Autodesk Inventor part; units mm, degrees
ref_plane "Work Plane1" through (0, 5, 0) normal (0, 1, 0) x (1, 0, 0)
ref_plane "YZ Plane" through (0, 0, 0) normal (1, 0, 0) x (0, 1, 0)
ref_plane "XZ Plane" through (0, 0, 0) normal (0, 1, 0) x (-1, 0, 0)
sketch "Sketch1" plane through (0, 0, 0) normal (0, 1, 0) x (-1, 0, 0)
  line L0 (0, -10) -> (-8.6603, -5)
  line L1 (-8.6603, -5) -> (-8.6603, 5)
  line L2 (-8.6603, 5) -> (0, 10)
  line L3 (0, 10) -> (8.6603, 5)
  line L4 (8.6603, 5) -> (8.6603, -5)
  line L5 (8.6603, -5) -> (0, -10)
  point P0 (0, 0)
  point P1 (0, 0)
  dimension "d1" = 20
extrude "Extrusion1" add sketch "Sketch1" along normal blind 10
sketch "Sketch2" plane through (0, 0, 0) normal (1, 0, 0) x (0, 1, 0)
  line L0 (10, -5) -> (10, -10)
  line L1 (10, -10) -> (8.5, -10)
  line L2 (10, -8.5) -> (10, -10)
  line L3 (8.5, -10) -> (10, -8.5)
  line L4 (-2, 0) -> (12, 0)
  point P0 (0, 0)
revolve "Revolution1" cut sketch "Sketch2" angle 360 about axis through (0, -10, 0) along (0, 1, 0)
ref_plane "Work Plane1" through (0, 5, 0) normal (0, 1, 0) x (1, 0, 0)
mirror "Mirror1" about plane through (0, 5, 0) normal (0, 1, 0) of "Revolution1"
sketch "Sketch3" plane through (0, 10, 0) normal (0, 1, 0) x (1, 0, 0)
  circle A0 centre (0, 0) radius 8.5
hole "Hole1" at (0, 10, 0) direction (0, -1, 0) diameter 10.917 depth 29.1 tip angle 118
chamfer "Chamfer1" distance 0.5 angle 45 2 edges at (0, 10, -5.4585) (0, 0, -5.4585)
properties part number "nut"
Could you check a few things on this model? Use its own coordinates, in mm. Give positions to 0.01 mm unless a question says otherwise; leave off trailing zeros. Order: outer loops, then holes, each group sorted by start corner. A loop starts at its lowest first (then second) coordinate and runs counter-clockwise, first axis right, second up. Notation, with made-up numbers: (83.25, 70) -> (117.25, 70) arc R28 cw to (117.25, 109) -> close; hole circle Ø2 at (43, -31). An arc over 180 degrees is marked (long way). Return JSON: item names as keys, results as strings.
1. Imagine slicing it at B-B on y = 7.5. List the corners of the cut face in (x, z) for me.
Answer list:
{"outline": "(-8.66, -5) -> (0, -10) -> (8.66, -5) -> (8.66, 5) -> (0, 10) -> (-8.66, 5) -> close; hole circle Ø10.92 at (0, 0)"}
2. Thinking about a two-plate mould opening in Z: for faces 1 (the flat face through (-4.27, 4.932, 7.535)), 2 (the cylindrical face through (5.33, 4.94, -1.18)), 3 (the flat face through (-2, 0, 6)), 4 (the flat face through (-4.391, 4.932, -7.465)), which applies, pulls with the +Z half, pulls with the -Z half, needs draft (parallel to the pull), parting line crosses it, or undercut?
Answer list:
{"face 1": "pulls with the +Z half", "face 2": "undercut", "face 3": "needs draft", "face 4": "pulls with the -Z half"}
3. For pin 1 Ø2 at (y, z) = (9, 6) entering from +X; pin 2 Ø4 at (x, y) = (0.5, 5.5) entering from +Z; pin 3 Ø3 at (x, y) = (0, 5) entering from -Z, each with a flat end and sliding along its axis, tell me the tip position at first contact or that it passes through.
Answer list:
{"pin 1": "stops at x = 8.51", "pin 2": "stops at z = 10", "pin 3": "stops at z = -10"}
4. I need wall thicknesses on line 1 (X direction, y = 4.25, z = 0); line 2 (X direction, y = 5, z = 1); line 3 (Z direction, x = 7, y = 7.25). Which ranges of each line are inside material? Lowest first, please. Write a range as from..to.
Answer list:
{"line 1": "x = -8.66..-5.46, 5.46..8.66", "line 2": "x = -8.66..-5.37, 5.37..8.66", "line 3": "z = -5.96..5.96"}
5. Imagine slicing it at A-A on z = 0. List the corners of the cut face in (x, y) for me, then the cut area to 3 significant figures.
Answer list:
{"outline": "(-8.66, 0.16) -> (-8.5, 0) -> (-5.96, 0) -> (-5.46, 0.5) -> (-5.46, 9.5) -> (-5.96, 10) -> (-8.5, 10) -> (-8.66, 9.84) -> close; (5.46, 0.5) -> (5.96, 0) -> (8.5, 0) -> (8.66, 0.16) -> (8.66, 9.84) -> (8.5, 10) -> (5.96, 10) -> (5.46, 9.5) -> close", "area": "63.5 mm2"}
